```python
from build123d import *

# Parameters (mm, degrees)
SKETCH_1_R      = 1.5
EXTRUDE_1_DEPTH = 1.2
SKETCH_2_W      = 13.910579459
SKETCH_2_H      = 13.201638929
SKETCH_2_H_2    = 13.209823538
SKETCH_2_H_3    = 4.905965234
EXTRUDE_2_DEPTH = 10
SKETCH_3_W      = 43.193790083
SKETCH_3_H      = 6.962206473
EXTRUDE_3_DEPTH = 10


with BuildPart() as part:
    # 草图1 → 凸台-拉伸1 (new body)
    with BuildSketch(Plane(origin=(0, 0, 0), x_dir=(1, 0, 0), z_dir=(0, 1, 0))):
        with BuildLine():
            Line((48, -31), (-48, -31))
            ThreePointArc((-48, -31), (-49.414213562, -30.414213562), (-50, -29))
            Line((-50, -29), (-50, 29))
            ThreePointArc((-50, 29), (-49.414213562, 30.414213562), (-48, 31))
            Line((-48, 31), (48, 31))
            ThreePointArc((48, 31), (49.414213562, 30.414213562), (50, 29))
            Line((50, 29), (50, -29))
            ThreePointArc((50, -29), (49.414213562, -30.414213562), (48, -31))
        make_face()
        with Locations(Location((-47, 28, 0), (0, 0, 270))):
            Circle(SKETCH_1_R, mode=Mode.SUBTRACT)
        with Locations(Location((47, 28, 0), (0, 0, 270))):
            Circle(SKETCH_1_R, mode=Mode.SUBTRACT)
        with Locations(Location((47, -28, 0), (0, 0, 270))):
            Circle(SKETCH_1_R, mode=Mode.SUBTRACT)
        with Locations(Location((-47, -28, 0), (0, 0, 270))):
            Circle(SKETCH_1_R, mode=Mode.SUBTRACT)
    extrude(amount=EXTRUDE_1_DEPTH)

    # 草图2 → 凸台-拉伸2 (add)
    with BuildSketch(Plane(origin=(0, 1.2, 0), x_dir=(1, 0, 0), z_dir=(0, 1, 0))):
        with Locations((-43.044710271, -13.054661049)):
            Rectangle(SKETCH_2_W, SKETCH_2_H)
        with Locations((-43.044710271, 3.320886699)):
            Rectangle(SKETCH_2_W, SKETCH_2_H_2)
        with Locations((-43.044710271, 15.810299107)):
            Rectangle(SKETCH_2_W, SKETCH_2_H_3)
    extrude(amount=EXTRUDE_2_DEPTH)

    # 草图3 → 凸台-拉伸3 (add)
    with BuildSketch(Plane(origin=(0, 1.2, 0), x_dir=(1, 0, 0), z_dir=(0, 1, 0))):
        with Locations((21.596895042, -26.824460666)):
            Rectangle(SKETCH_3_W, SKETCH_3_H)
    extrude(amount=EXTRUDE_3_DEPTH)


solid = part.part
```
Input: part model. Units: mm. Frame: model coordinates. A direction names the side the tool comes from. Coordinates: 2 decimals unless noted, no trailing zeros. Loops run counter-clockwise (first coordinate to the right, second up) from the corner with the lowest first, then second, coordinate; pieces in that order, holes last. Notation, with made-up numbers: M 82,70.25 L 121,70.25 A9 cw 121,82.25 Z; hole C 76.25,40.5 d3. An arc over 180 degrees is marked long. One line per item, written item: value.
(1) Pin query (flat end, axial travel): pin 1 (3 mm diameter, centred on x = -42.5, y = 8.5, fed in from +Z); pin 2 (6 mm diameter, centred on x = -39, z = -21.5, fed in from -Y); pin 3 (3.5 mm diameter, centred on x = 47, z = -28, fed in from +Y); pin 4 (4 mm diameter, centred on y = 4.5, z = -16, fed in from +X). Return the tip coordinate at first contact, or that it passes through.
Filled in:
pin 1: z = 19.66
pin 2: y = 0
pin 3: y = 1.2
pin 4: x = -36.09
(2) Pull-direction query (Z, two-part tool) for faces 4 (the flat face through (1, 0, 0)), 5 (the cylindrical face through (-48.464, 0.592, -28.325)), 6 (the flat face through (-43, 6, -18.263)); classes: +Z half, -Z half, draft (parallel to the pull), parting line (faces both ways), or undercut.
Filled in:
face 4: draft
face 5: undercut
face 6: -Z half
(3) Section B-B (x = -47). Output: boundary loops of the cut face in (y, z), and give its area (3 significant figures).
Filled in:
outline: M 0,-31 L 1.2,-31 L 1.2,-29.5 L 0,-29.5 Z; M 0,-26.5 L 1.2,-26.5 L 1.2,-18.26 L 11.2,-18.26 L 11.2,-13.36 L 1.2,-13.36 L 1.2,-9.93 L 11.2,-9.93 L 11.2,3.28 L 1.2,3.28 L 1.2,6.45 L 11.2,6.45 L 11.2,19.66 L 1.2,19.66 L 1.2,26.5 L 0,26.5 Z; M 0,29.5 L 1.2,29.5 L 1.2,31 L 0,31 Z
area: 380 mm^2
(4) Section C-C (y = 5.75). Output: boundary loops of the cut face in (x, z), and give its area (3 significant figures).
Filled in:
outline: M -50,-18.26 L -36.09,-18.26 L -36.09,-13.36 L -50,-13.36 Z; M -50,-9.93 L -36.09,-9.93 L -36.09,3.28 L -50,3.28 Z; M -50,6.45 L -36.09,6.45 L -36.09,19.66 L -50,19.66 Z; M 0,23.34 L 43.19,23.34 L 43.19,30.31 L 0,30.31 Z
area: 736 mm^2
(5) Section A-A (z = -28). Output: boundary loops of the cut face in (x, y).
Filled in:
outline: M -50,0 L -48.5,0 L -48.5,1.2 L -50,1.2 Z; M -45.5,0 L 45.5,0 L 45.5,1.2 L -45.5,1.2 Z; M 48.5,0 L 50,0 L 50,1.2 L 48.5,1.2 Z
(6) Section D-D (x = 1). Output: boundary loops of the cut face in (y, z), and give its area (3 significant figures).
Filled in:
outline: M 0,-31 L 1.2,-31 L 1.2,23.34 L 11.2,23.34 L 11.2,30.31 L 1.2,30.31 L 1.2,31 L 0,31 Z
area: 144 mm^2
(7) Reachability of faces 1 (the flat face through (-36.089, 6, 13)), 2 (the flat face through (21, 11.2, 27)), 3 (the flat face through (-43, 6, 6.454)) from +Z, -Z, +X, -X, +Y, -Y: full face, straight path, thin tool, end or side. Return the list, or none.
Filled in:
face 1: +Z, -Z, +X, +Y
face 2: +Z, -Z, +X, -X, +Y
face 3: +X, -X, +Y
(8) Line query: line 1 along X through (y, z) = (0.5, -28); line 2 along Z through (x, y) = (-36.5, 7.5); line 3 along Y through (x, z) = (-10, 13). Output: solid intervals per line, ascending. Write a range as from..to.
Filled in:
line 1: -50..-48.5, -45.5..45.5, 48.5..50
line 2: -18.26..-13.36, -9.93..3.28, 6.45..19.66
line 3: 0..1.2
